For this review, use the dimensioned drawing (mm, ordinates from the lowest corner) and the shaded views. A direction names the side the tool comes from. Coordinates: 2 decimals unless noted, no trailing zeros. Loops run counter-clockwise (first coordinate to the right, second up) from the corner with the lowest first, then second, coordinate; pieces in that order, holes last. Notation, with made-up numbers: M 12.25,16.25 L 28.25,16.25 A7 ccw 28.25,27.25 Z; hole C 67,15 d6. An arc over 180 degrees is marked long. One line per item, written item: value.
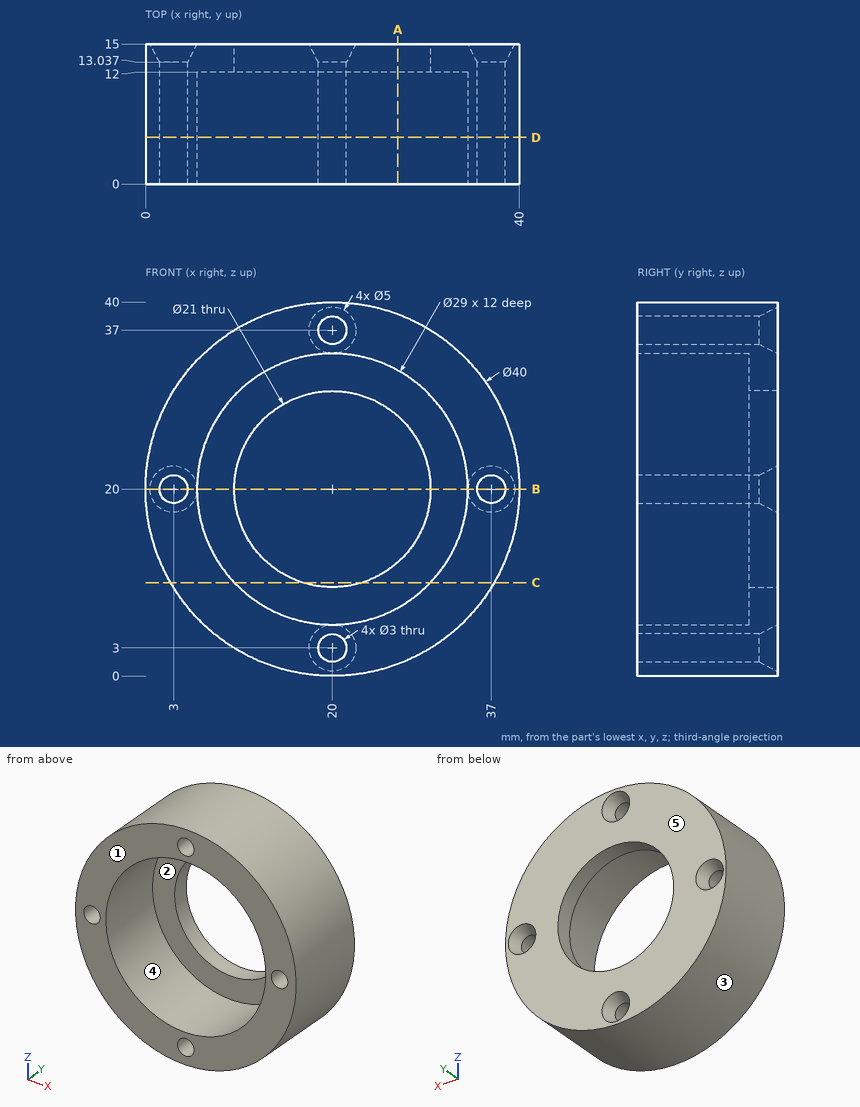
(1) Add section A-A on x = 27. State the section outline as (y, z) points (1 decimal), then the cut area to 3 significant figures.
Checks:
outline: M 0,1.3 L 15,1.3 L 15,12.2 L 12,12.2 L 12,7.3 L 0,7.3 Z; M 0,32.7 L 12,32.7 L 12,27.8 L 15,27.8 L 15,38.7 L 0,38.7 Z
area: 210 mm^2
(2) Tool access review of the marked faces 1 and 2: name each direction out of +Z, -Z, +X, -X, +Y, -Y from which nothing blocks a thin tool from reaching the whole face with its end or side.
Checks:
face 1: +Z, -Z, +X, -X, -Y
face 2: -Y
(3) Draft analysis for pull direction X (two halves, no side actions). For the marked faces 3, 4 and 5, state which applies: pulls with the +X half, pulls with the -X half, needs draft (parallel to the pull), parting line crosses it, or undercut.
Checks:
face 3: parting line crosses it
face 4: undercut
face 5: needs draft
(4) Add section D-D on y = 5. State the section outline as (x, z) points.
Checks:
outline: C 20,20 d40; hole C 3,20 d3; hole C 20,20 d29; hole C 20,3 d3; hole C 20,37 d3; hole C 37,20 d3
(5) Add section C-C on z = 10. State the section outline as (x, y) points.
Checks:
outline: M 2.68,0 L 9.5,0 L 9.5,12 L 16.8,12 L 16.8,15 L 2.68,15 Z; M 23.2,12 L 30.5,12 L 30.5,0 L 37.32,0 L 37.32,15 L 23.2,15 Z
(6) Insertion check: pin 1 Ø6 at (y, z) = (13.5, 34) entering from -X; pin 2 Ø2 at (y, z) = (10, 23) entering from -X; pin 3 Ø4 at (x, z) = (3, 20) entering from +Y. Each pin has a flat end and moves straight along its axis. Give the tip position at first contact, or say it passes through.
Checks:
pin 1: x = 3.3
pin 2: x = 0.1
pin 3: y = 14.02
(7) Add section B-B on z = 20. State the section outline as (x, y) points.
Checks:
outline: M 0,0 L 1.5,0 L 1.5,13.04 L 0.5,15 L 0,15 Z; M 4.5,0 L 5.5,0 L 5.5,12 L 9.5,12 L 9.5,15 L 5.5,15 L 4.5,13.04 Z; M 30.5,12 L 34.5,12 L 34.5,0 L 35.5,0 L 35.5,13.04 L 34.5,15 L 30.5,15 Z; M 38.5,0 L 40,0 L 40,15 L 39.5,15 L 38.5,13.04 Z
(8) To check wall thickness, follow L1, parallel to X at y = 8.75, z = 20; L2, parallel to Z at x = 3, y = 3.5 (1 decimal); L3, parallel to Z at x = 2.5, y = 9.25 (1 decimal). State the ranges of each line that lie inside material, in increasing order. Write a range as [from, to].
Checks:
L1: [0, 1.5], [4.5, 5.5], [34.5, 35.5], [38.5, 40]
L2: [9.5, 18.5], [21.5, 30.5]
L3: [10.3, 18.6], [21.4, 29.7]
